Geometry: final body of the model. Coordinates: model frame, mm. A direction names the side the tool comes from. Give positions to 0.01 mm unless a question says otherwise; leave off trailing zeros. Write each loop counter-clockwise with the first axis right and the second up, starting at its lowest first coordinate (ties: lowest second). Pieces come first, ordered by that corner, then holes. Notation, with made-up numbers: (-35.5, 57) -> (-29.5, 57) arc R24 cw to (-29.5, 72) -> close; hole circle Ø3 at (58, 33.25). An arc over 180 degrees is marked (long way). Answer as a JSON object with one key per item and string values.
from build123d import *

# Parameters (mm, degrees)
F0_R     = 10
F1_DEPTH = 675
F2_SIZE  = 2
F4_W     = 21
F4_H     = 15
F5_DEPTH = 1.5


with BuildPart() as f1:
    # F0 (on Top) → F1 (new body)
    with BuildSketch(Plane.XY):
        Circle(F0_R)
    extrude(amount=F1_DEPTH)

    # F2
    f2_edges = [f1.edges().sort_by_distance(p)[0] for p in [
        (-10, 0, 0),
        (-10, 0, 675),
    ]]
    chamfer(f2_edges, length=F2_SIZE)

    # F4 (on offset) → F5 (cut)
    with BuildSketch(Plane.YZ.offset(10)):
        with Locations((0, 7.5)):
            Rectangle(F4_W, F4_H)
    extrude(amount=-F5_DEPTH, mode=Mode.SUBTRACT)


solid = f1.part
Q1. First-contact query: P1, Ø10, axis at y = -0.5, z = 485.5, coming from the -X side; P2, Ø3, axis at y = 1, z = 9, coming from the +X side; P3, Ø5, axis at y = -5, z = 502, coming from the -X side; P4, Ø1, axis at x = 7.5, z = 490, coming from the +Y side. Flat tips, straight axial feed; report the tip coordinate or a pass-through.
Values:
{"P1": "x = -10", "P2": "x = 8.5", "P3": "x = -9.68", "P4": "y = 7.14"}
Q2. Material intervals for L1, parallel to Y at x = -0.25, z = 408; L2, parallel to Y at x = 1.25, z = 60; L3, parallel to X at y = 6, z = 552, sorted ascending. Write a range as from..to.
Values:
{"L1": "-10..10", "L2": "-9.92..9.92", "L3": "-8..8"}
Q3. Set-up query: faces 1 (the flat face through (0, 0, 0)), 2 (the flat face through (8.5, 0, 8)). Return all of +Z, -Z, +X, -X, +Y, -Y with unobstructed straight access to the full face (end or side cutting, diameter ignored); none if empty.
Values:
{"face 1": "-Z, +X, -X, +Y, -Y", "face 2": "-Z, +X, +Y, -Y"}
Q4. Cut plane A-A (z = 383). Return the cut outline in (x, y).
Values:
{"outline": "circle Ø20 at (0, 0)"}
